Autodesk Inventor part; units mm, degrees
ref_plane "Work Plane1" through (0, 0, 0) normal (0, 0, 1) x (1, 0, 0)
ref_plane "YZ Plane" through (0, 0, 0) normal (1, 0, 0) x (0, 1, 0)
ref_plane "XZ Plane" through (0, 0, 0) normal (0, 1, 0) x (-1, 0, 0)
ref_plane "Work Plane1" through (0, 0, 0) normal (0, 0, 1) x (1, 0, 0)
sketch "Sketch1" plane through (0, 0, 0) normal (0, 0, 1) x (1, 0, 0)
  line L0 (302, -174.3598) -> (0, -348.7196)
  line L1 (0, -348.7196) -> (-302, -174.3598)
  line L2 (-302, -174.3598) -> (-302, 174.3598)
  line L3 (-302, 174.3598) -> (0, 348.7196)
  line L4 (0, 348.7196) -> (302, 174.3598)
  line L5 (302, 174.3598) -> (302, -174.3598)
  line L6 (498, -287.5204) -> (0, -575.0409)
  line L7 (0, -575.0409) -> (-498, -287.5204)
  line L8 (-498, -287.5204) -> (-498, 287.5204)
  line L9 (-498, 287.5204) -> (0, 575.0409)
  line L10 (0, 575.0409) -> (498, 287.5204)
  line L11 (498, 287.5204) -> (498, -287.5204)
  point P0 (0, 0)
  point P1 (0, 0)
  point P2 (0, 0)
  dimension "d0" = 302
  dimension "d1" = 498
extrude "Extrusion1" add sketch "Sketch1" along normal blind 50
properties part number "Sustrat"
Geometry: final body of the model. Coordinates: model frame, mm. A direction names the side the tool comes from. Give positions to 0.01 mm unless a question says otherwise; leave off trailing zeros. Loops run counter-clockwise (first coordinate to the right, second up) from the corner with the lowest first, then second, coordinate; pieces in that order, holes last. Notation, with made-up numbers: (-32, 72) -> (10, 72) arc R11 ccw to (10, 78) -> close; hole circle Ø1 at (17, -15). An arc over 180 degrees is marked (long way). Use CSV: the item, a comma, the result in double quotes.
(1) Cut plane A-A (y = 140). Output: boundary loops of the cut face in (x, z).
From the geometry:
outline,"(-498, 0) -> (-302, 0) -> (-302, 50) -> (-498, 50) -> close; (302, 0) -> (498, 0) -> (498, 50) -> (302, 50) -> close"
(2) Access query for faces 1 (the face through (245.5, 433.3, 24.6)), 2 (the face through (302, 2, 25)). Directions: +Z, -Z, +X, -X, +Y, -Y. A direction counts if a zero-diameter tool reaches every point of the face in a straight line with its end or side. Return the directions, or none.
From the geometry:
face 1,"+Z, -Z, +X, +Y"
face 2,"+Z, -Z"
(3) Ray query, line 1 along X through (y, z) = (92, 30); line 2 along X through (y, z) = (304, 44.5); line 3 along Y through (x, z) = (279.5, 25). Return the intervals inside material, ascending. Write a range as [from, to].
From the geometry:
line 1,"[-498, -302], [302, 498]"
line 2,"[-469.46, -77.46], [77.46, 469.46]"
line 3,"[-413.67, -187.35], [187.35, 413.67]"
(4) Pull-direction query (Y, two-part tool) for faces 3 (the face through (-252.486, 429.268, 24.65)), 4 (the face through (-498, -4, 25)), 5 (the face through (-148.89, -262.76, 24.65)); classes: released by +Y, released by -Y, zero draft, split by the parting line, or undercut.
From the geometry:
face 3,"released by +Y"
face 4,"zero draft"
face 5,"undercut"
(5) Cut plane D-D (y = -415.5). Output: boundary loops of the cut face in (x, z), plus the area to 3 significant figures.
From the geometry:
outline,"(-276.33, 0) -> (276.33, 0) -> (276.33, 50) -> (-276.33, 50) -> close"
area,"27,600 mm^2"
(6) First-contact query: P1, Ø2, axis at x = -285.5, y = 318.5, coming from the -Z side; P2, Ø3, axis at x = 179, z = 24, coming from the -Y side; P3, Ø5, axis at x = -49.5, z = 36, coming from the -Y side. Flat tips, straight axial feed; report the tip coordinate or a pass-through.
From the geometry:
P1,"z = 0"
P2,"y = -472.56"
P3,"y = -547.91"
(7) Cut plane C-C (x = 162). Output: boundary loops of the cut face in (y, z), plus the area to 3 significant figures.
From the geometry:
outline,"(-481.51, 0) -> (-255.19, 0) -> (-255.19, 50) -> (-481.51, 50) -> close; (255.19, 0) -> (481.51, 0) -> (481.51, 50) -> (255.19, 50) -> close"
area,"22,600 mm^2"
(8) Cut plane B-B (z = 9). Output: boundary loops of the cut face in (x, y).
From the geometry:
outline,"(-498, -287.52) -> (0, -575.04) -> (498, -287.52) -> (498, 287.52) -> (0, 575.04) -> (-498, 287.52) -> close; hole (-302, -174.36) -> (0, -348.72) -> (302, -174.36) -> (302, 174.36) -> (0, 348.72) -> (-302, 174.36) -> close"
